```python
from build123d import *

# Parameters (mm, degrees)
MEPLATFIXING_DEPTH                 = 3
MEPLATROTOR_DEPTH                  = 15
ESQUISSE4_R                        = 1.5
FIXINGHOLE_DEPTH                   = 5
FIXINGHOLECIRCULARREPETITION_COUNT = 4


with BuildPart() as part:
    # Esquisse1 → Révolution1 (revolve)
    with BuildSketch(Plane.XY):
        Polygon((-38, 13.75), (0, 13.75), (0, 16), (33.5, 16), (33.5, 10), (36.5, 10), (36.5, 3), (51.5, 3), (51.5, 0), (-38, 0), align=None)
    revolve(axis=Axis((-42.475, 0, 0), (1, 0, 0)))

    # Esquisse2 → MeplatFixing (cut)
    with BuildSketch(Plane(origin=(36.5, 0, 0), x_dir=(0, 0, -1), z_dir=(1, 0, 0))):
        with BuildLine():
            Line((-4.358898944, 9), (4.358898944, 9))
            ThreePointArc((4.358898944, 9), (0, 10), (-4.358898944, 9))
        make_face()
        with BuildLine():
            Line((-4.358898944, -9), (4.358898944, -9))
            ThreePointArc((4.358898944, -9), (0, -10), (-4.358898944, -9))
        make_face()
    extrude(amount=-MEPLATFIXING_DEPTH, mode=Mode.SUBTRACT)

    # Esquisse3 → MeplatRotor (cut)
    with BuildSketch(Plane(origin=(51.5, 0, 0), x_dir=(0, 0, -1), z_dir=(1, 0, 0))):
        with BuildLine():
            Line((-1.658312395, 2.5), (1.658312395, 2.5))
            ThreePointArc((1.658312395, 2.5), (0, 3), (-1.658312395, 2.5))
        make_face()
    extrude(amount=-MEPLATROTOR_DEPTH, mode=Mode.SUBTRACT)

    # Esquisse4 → FixingHole (cut)
    with BuildSketch(Plane(origin=(33.5, 0, 0), x_dir=(0, 0, -1), z_dir=(1, 0, 0))):
        with Locations((9.192388155, 9.192388155)):
            Circle(ESQUISSE4_R)
    fixinghole = extrude(amount=-FIXINGHOLE_DEPTH, mode=Mode.SUBTRACT)

    # FixingHoleCircularRepetition: FixingHole ×4 about axis
    fixingholecircularrepetition_axis = Axis((0, 0, 0), (1, 0, 0))
    for i in range(1, FIXINGHOLECIRCULARREPETITION_COUNT):
        add(fixinghole.rotate(fixingholecircularrepetition_axis, i * 360 / FIXINGHOLECIRCULARREPETITION_COUNT), mode=Mode.SUBTRACT)


solid = part.part
```
Geometry: final body of the model. Coordinates: model frame, mm. A direction names the side the tool comes from. Coordinates: 2 decimals unless noted, no trailing zeros. Write each loop counter-clockwise with the first axis right and the second up, starting at its lowest first coordinate (ties: lowest second). Pieces come first, ordered by that corner, then holes. Notation, with made-up numbers: M -11.75,0.25 L 15.25,0.25 A26 ccw 15.25,31.25 Z; hole C 79,61 d3. An arc over 180 degrees is marked long. Answer as CSV lines item,"result". Start each with the question number.
Q1. Mould query, pull axis Z, two halves, no side actions, for faces 6 (the cylindrical face through (31.04, -8.28, 8)), 7 (the cylindrical face through (-18.734, -2.981, -13.423)), 8 (the cylindrical face through (35, 0, -10)), 9 (the flat face through (35, 9, 0)). Classes: released by +Z, released by -Z, zero draft, split by the parting line, or undercut.
Q2. Cut plane A-A on y = 0. Return the cut outline in (x, z), then the cut area to 3 significant figures.
Q3. Reachability of faces 1 (the flat face through (0, -5, 13)), 2 (the flat face through (33.5, -0.2, -10.4)), 3 (the flat face through (35, -9, 0)), 4 (the flat face through (44, 2.5, 0)), 5 (the flat face through (-38, 0, 0)) from +Z, -Z, +X, -X, +Y, -Y: full face, straight path, thin tool, end or side. Return the list, or none.
Q4. Cut plane C-C on z = 0. Return the cut outline in (x, y).
Q5. Pin query (flat end, axial travel): P1, Ø4, axis at x = 42.5, y = -3.5, coming from the +Z side; P2, Ø3, axis at x = -1, z = 6.5, coming from the +Y side; P3, Ø2.5, axis at y = -10, z = -8.5, coming from the +X side. Return the tip coordinate at first contact, or that it passes through.
Q6. Cut plane D-D on x = 5.5. Return the cut outline in (y, z).
Q7. Line query: line 1 (X direction, y = 13, z = -1); line 2 (X direction, y = -0.5, z = 9); line 3 (Y direction, x = -8, z = 12). Output: solid intervals per line, ascending. Write a range as from..to.
Q8. Cut plane B-B on x = 32.5. Return the cut outline in (y, z), then the cut area to 3 significant figures.
Findings below:
1,face 6,"undercut"
1,face 7,"split by the parting line"
1,face 8,"released by -Z"
1,face 9,"zero draft"
2,outline,"M -38,-13.75 L 0,-13.75 L 0,-16 L 33.5,-16 L 33.5,-10 L 36.5,-10 L 36.5,-3 L 51.5,-3 L 51.5,3 L 36.5,3 L 36.5,10 L 33.5,10 L 33.5,16 L 0,16 L 0,13.75 L -38,13.75 Z"
2,area,"2,270 mm2"
3,face 1,"-X"
3,face 2,"+X"
3,face 3,"+Z, -Z, +X, -Y"
3,face 4,"+Z, -Z, +X, +Y"
3,face 5,"+Z, -Z, -X, +Y, -Y"
4,outline,"M -38,-13.75 L 0,-13.75 L 0,-16 L 33.5,-16 L 33.5,-9 L 36.5,-9 L 36.5,-3 L 51.5,-3 L 51.5,2.5 L 36.5,2.5 L 36.5,9 L 33.5,9 L 33.5,16 L 0,16 L 0,13.75 L -38,13.75 Z"
5,P1,"stops at z = 2.6"
5,P2,"stops at y = 15.07"
5,P3,"stops at x = 33.5"
6,outline,"C 0,0 d32"
7,line 1,"x = -38..33.5"
7,line 2,"x = -38..36.5"
7,line 3,"y = -6.71..6.71"
8,outline,"C 0,0 d32; hole C -9.19,-9.19 d3; hole C -9.19,9.19 d3; hole C 9.19,-9.19 d3; hole C 9.19,9.19 d3"
8,area,"776 mm2"
